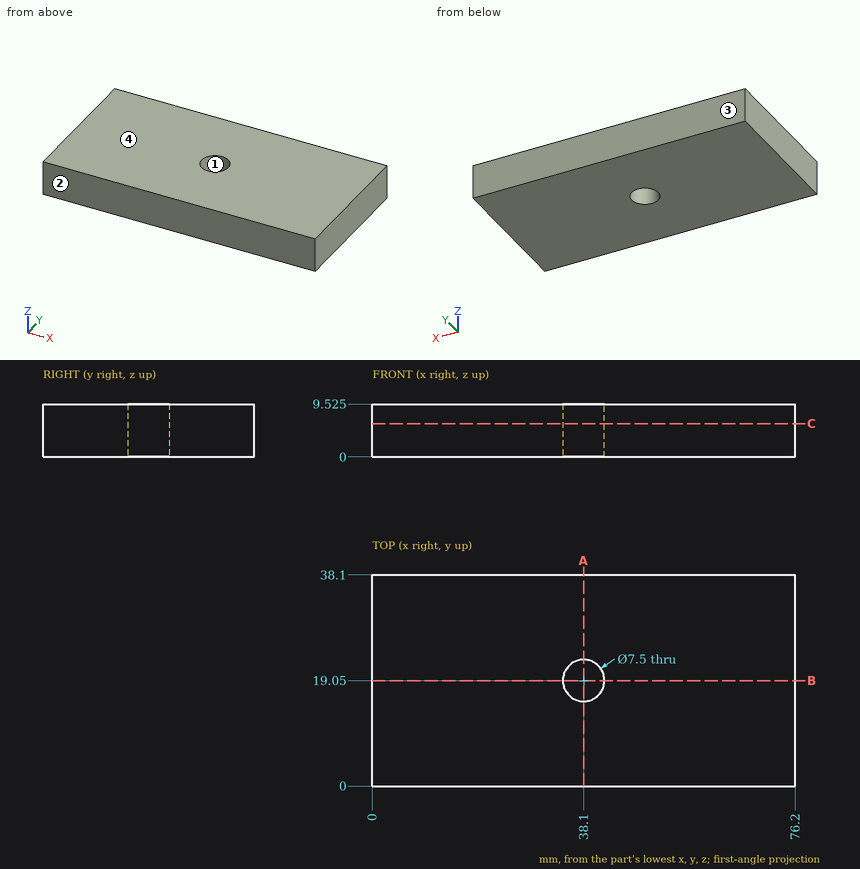
Geometry: see drawing. Coordinates: mm, zero at the bounding-box minimum. Give positions to 0.01 mm unless a question says otherwise; leave off trailing zeros. Loops run counter-clockwise (first coordinate to the right, second up) from the corner with the lowest first, then second, coordinate; pieces in that order, holes last. Notation, with made-up numbers: (-29, 32.5) -> (10, 32.5) arc R18 cw to (10, 55.5) -> close; hole circle Ø11 at (-11.5, 68). An arc over 180 degrees is marked (long way). Use CSV: the item, a comma, the result in double quotes.
(1) Cut plane C-C (z = 6). Output: boundary loops of the cut face in (x, y).
From the geometry:
outline,"(0, 0) -> (76.2, 0) -> (76.2, 38.1) -> (0, 38.1) -> close; hole circle Ø7.5 at (38.1, 19.05)"
(2) Cut plane B-B (y = 19.05). Output: boundary loops of the cut face in (x, z) (3 decimals).
From the geometry:
outline,"(0, 0) -> (34.35, 0) -> (34.35, 9.525) -> (0, 9.525) -> close; (41.85, 0) -> (76.2, 0) -> (76.2, 9.525) -> (41.85, 9.525) -> close"
(3) Pull-direction query (Y, two-part tool) for the marked faces 1, 2, 3 and 4; classes: released by +Y, released by -Y, zero draft, split by the parting line, or undercut.
From the geometry:
face 1,"undercut"
face 2,"released by -Y"
face 3,"released by +Y"
face 4,"zero draft"
(4) Ray query, line 1 along Y through (x, z) = (38.1, 4.75); line 2 along X through (y, z) = (21.5, 5.25); line 3 along Y through (x, z) = (36.5, 0.75). Return the intervals inside material, ascending. Write a range as [from, to].
From the geometry:
line 1,"[0, 15.3], [22.8, 38.1]"
line 2,"[0, 35.26], [40.94, 76.2]"
line 3,"[0, 15.66], [22.44, 38.1]"
(5) Cut plane A-A (x = 38.1). Output: boundary loops of the cut face in (y, z) (3 decimals).
From the geometry:
outline,"(0, 0) -> (15.3, 0) -> (15.3, 9.525) -> (0, 9.525) -> close; (22.8, 0) -> (38.1, 0) -> (38.1, 9.525) -> (22.8, 9.525) -> close"
